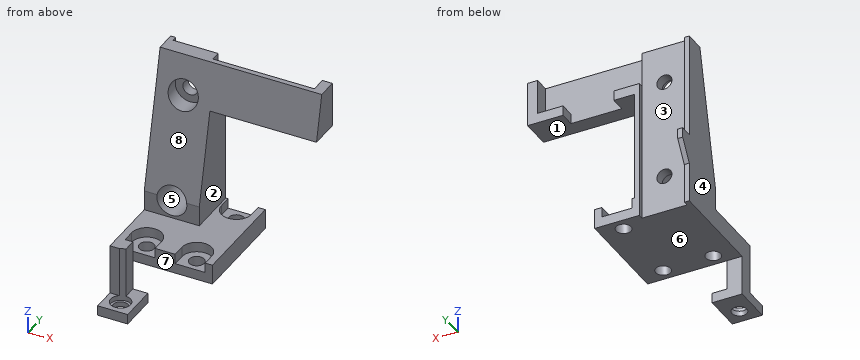
from build123d import *

# Parameters (mm, degrees)
SKETCH_W        = 18.9
SKETCH_H        = 20
SKETCH_R        = 1.5
PAD_DEPTH       = 8
SKETCH001_W     = 3
SKETCH001_H     = 16
PAD001_DEPTH    = 3
SKETCH002_W     = 6
SKETCH002_H     = 7.65
SKETCH002_R     = 1.5
PAD002_DEPTH    = 2
SKETCH003_R     = 2
POCKET_DEPTH    = 15
PAD003_DEPTH    = 10
SKETCH005_R     = 1.5
POCKET001_DEPTH = 10
SKETCH006_W     = 9
SKETCH006_H     = 35
POCKET002_DEPTH = 1
POCKET003_DEPTH = 3
SKETCH008_W     = 1
SKETCH008_H     = 6.05
PAD004_DEPTH    = 2.5
POCKET004_DEPTH = 32.301
POCKET005_DEPTH = 32.301
POCKET014_DEPTH = 6
POCKET015_DEPTH = 4
SKETCH023_R     = 3
POCKET017_DEPTH = 8


with BuildPart() as part:
    # Sketch (on Face6 of Binder) → Pad (new body)
    with BuildSketch(Plane.XY.offset(8)):
        with Locations((14.45, 10)):
            Rectangle(SKETCH_W, SKETCH_H)
        with Locations((19.45, 17.5)):
            Circle(SKETCH_R, mode=Mode.SUBTRACT)
        with Locations((9.45, 2.5)):
            Circle(SKETCH_R, mode=Mode.SUBTRACT)
        with Locations((19.45, 2.5)):
            Circle(SKETCH_R, mode=Mode.SUBTRACT)
    extrude(amount=PAD_DEPTH)

    # Sketch001 (on Face3 of Pad) → Pad001 (join)
    with BuildSketch(Plane.XZ):
        with Locations((6.5, 8)):
            Rectangle(SKETCH001_W, SKETCH001_H)
    extrude(amount=PAD001_DEPTH)

    # Sketch002 (on Face13 of Pad001) → Pad002 (join)
    with BuildSketch(Plane(origin=(0, 0, 0), x_dir=(1, 0, 0), z_dir=(0, 0, -1))):
        with Locations((8, 3.825)):
            Rectangle(SKETCH002_W, SKETCH002_H)
        with Locations((8, 4.65)):
            Circle(SKETCH002_R, mode=Mode.SUBTRACT)
    extrude(amount=-PAD002_DEPTH)

    # Sketch003 (on Face12 of Pad002) → Pocket (cut)
    with BuildSketch(Plane.XY.offset(16)):
        with Locations((8, -4.65)):
            Circle(SKETCH003_R)
    extrude(amount=-POCKET_DEPTH, mode=Mode.SUBTRACT)

    # Sketch004 (on Face1 of Pocket) → Pad003 (join)
    with BuildSketch(Plane(origin=(0, 20, 0), x_dir=(-1, 0, 0), z_dir=(0, 1, 0))):
        Polygon((-5, 16), (-16, 16), (-16, 34.02), (-37.3, 34.02), (-37.3, 43), (-16, 43), (-5, 43), align=None)
    extrude(amount=-PAD003_DEPTH)

    # Sketch005 (on Face5 of Pad003) → Pocket001 (cut)
    with BuildSketch(Plane(origin=(0, 20, 0), x_dir=(-1, 0, 0), z_dir=(0, 1, 0))):
        with Locations((-10.5, 15.5)):
            Circle(SKETCH005_R)
        with Locations((-10.5, 35.5)):
            Circle(SKETCH005_R)
    extrude(amount=-POCKET001_DEPTH, mode=Mode.SUBTRACT)

    # Sketch006 (on Face5 of Pocket001) → Pocket002 (cut)
    with BuildSketch(Plane(origin=(0, 20, 0), x_dir=(-1, 0, 0), z_dir=(0, 1, 0))):
        with Locations((-10.5, 25.5)):
            Rectangle(SKETCH006_W, SKETCH006_H)
    extrude(amount=-POCKET002_DEPTH, mode=Mode.SUBTRACT)

    # Sketch007 (on Face21 of Pocket002) → Pocket003 (cut)
    with BuildSketch(Plane(origin=(0, 20, 0), x_dir=(-1, 0, 0), z_dir=(0, 1, 0))):
        Polygon((-15, 43), (-35.3, 43), (-35.3, 36.02), (-30.23, 36.02), (-30.23, 34.02), (-20.07, 34.02), (-20.07, 36.02), (-15, 36.02), align=None)
    extrude(amount=-POCKET003_DEPTH, mode=Mode.SUBTRACT)

    # Sketch008 (on Face4 of Pocket003) → Pad004 (join)
    with BuildSketch(Plane(origin=(0, 20, 0), x_dir=(-1, 0, 0), z_dir=(0, 1, 0))):
        with Locations((-5.5, 19.025)):
            Rectangle(SKETCH008_W, SKETCH008_H)
    extrude(amount=PAD004_DEPTH)

    # Sketch009 (on Face18 of Pad004) → Pocket004 (cut, through all)
    with BuildSketch(Plane(origin=(5, 0, 0), x_dir=(0, -1, 0), z_dir=(-1, 0, 0))):
        Polygon((-22.5, 20.05), (-20, 16), (-22.5, 16), align=None)
    extrude(amount=-POCKET004_DEPTH, mode=Mode.SUBTRACT)

    # Sketch010 (on Face22 of Pocket004) → Pocket005 (cut, through all)
    with BuildSketch(Plane(origin=(5, 0, 0), x_dir=(0, -1, 0), z_dir=(-1, 0, 0))):
        Polygon((-10, 16), (-16, 43), (-10, 43), align=None)
    extrude(amount=-POCKET005_DEPTH, mode=Mode.SUBTRACT)

    # Sketch020 (on Face21 of Pocket005) → Pocket014 (cut)
    with BuildSketch(Plane.XY.offset(16)):
        with BuildLine():
            ThreePointArc((16.45, 17.499996), (19.45, 14.5), (22.45, 17.499996))
            Line((22.45, 17.499996), (22.45, 20))
            Line((22.45, 20), (16.45, 20))
            Line((16.45, 20), (16.45, 17.499996))
        make_face()
        with BuildLine():
            ThreePointArc((22.45, 2.5), (19.45, 5.5), (16.45, 2.5))
            Line((16.45, 0), (16.45, 2.5))
            Line((22.45, 0), (16.45, 0))
            Line((22.45, 2.5), (22.45, 0))
        make_face()
        with BuildLine():
            ThreePointArc((12.45, 2.5), (9.45, 5.5), (6.45, 2.5))
            Line((6.45, 2.5), (6.45, 0))
            Line((6.45, 0), (12.45, 0))
            Line((12.45, 0), (12.45, 2.5))
        make_face()
    extrude(amount=-POCKET014_DEPTH, mode=Mode.SUBTRACT)

    # Sketch021 (on Face21 of Pocket014) → Pocket015 (cut)
    with BuildSketch(Plane.XY.offset(16)):
        Polygon((23.9, 0), (23.9, 10), (23.9, 20), (16, 20), (16, 10), (5, 10), (5, 0), (5, -3), (8, -3), (8, 0), align=None)
    extrude(amount=-POCKET015_DEPTH, mode=Mode.SUBTRACT)

    # Sketch023 (on Face6 of Pocket015) → Pocket017 (cut)
    with BuildSketch(Plane(origin=(0, 9, 0), x_dir=(-1, 0, 0), z_dir=(0, 1, 0))):
        with Locations((-10.5, 15.5)):
            Circle(SKETCH023_R)
        with Locations((-10.5, 35.5)):
            Circle(SKETCH023_R)
    extrude(amount=POCKET017_DEPTH, mode=Mode.SUBTRACT)


solid = part.part
Work out the finished part from the listing and answer in its coordinate system (mm). Face numbers are marked on the shaded views. A direction names the side the tool comes from. Coordinates: 2 decimals unless noted, no trailing zeros. Write each loop counter-clockwise with the first axis right and the second up, starting at its lowest first coordinate (ties: lowest second). Pieces come first, ordered by that corner, then holes. Notation, with made-up numbers: M -14,-32 L -4,-32 A12 ccw -4,-13 Z; hole C 13.5,14 d10. An arc over 180 degrees is marked long. Write item = value, one per line.
1. Determine the mould class of the marked faces 1, 2, 3 and 4 for opening direction X: released by +X, released by -X, zero draft, split by the parting line, or undercut.
Solution:
face_1 = zero draft
face_2 = released by +X
face_3 = undercut
face_4 = released by -X
2. For the marked faces 5, 6, 7 and 8, determine the directions among +Z, -Z, +X, -X, +Y, -Y from which every point of the face is accessible in a straight line to the end or side of a thin tool.
Solution:
face_5 = -Y
face_6 = -Z, +X, -X, +Y
face_7 = +Z, +X, -Y
face_8 = +Z, +X, -X, -Y
3. The part is cut by section D-D (x = 34.5). Determine the outline of the cut face in (y, z), then the cut area to 3 significant figures.
Solution:
outline = M 14,34.02 L 20,34.02 L 20,36.02 L 17,36.02 L 17,43 L 16,43 Z
area = 23.9 mm2
4. The part is cut by section B-B (y = -4.65). Determine the outline of the cut face in (x, z), then the cut area to 3 significant figures.
Solution:
outline = M 5,0 L 6.5,0 L 6.5,1 L 6,1 L 6,2 L 5,2 Z; M 9.5,0 L 11,0 L 11,2 L 10,2 L 10,1 L 9.5,1 Z
area = 5.00 mm2
5. The part is cut by section C-C (z = 15.5). Determine the outline of the cut face in (x, y).
Solution:
outline = M 5,10 L 7.5,10 L 7.5,17 L 9,17 L 9,19 L 6,19 L 6,20 L 5,20 Z; M 12,17 L 13.5,17 L 13.5,10 L 16,10 L 16,20 L 15,20 L 15,19 L 12,19 Z
6. Straight lines are drawn through the part: line 1 (Z direction, x = 10.5, y = 18.5); line 2 (Y direction, x = 19.45, z = 9.05); line 3 (X direction, y = -4.65, z = 0.6). For each, find the intervals that lie inside material, in ascending order. Write a range as from..to.
Solution:
line_1 = 8..14, 17..34, 37..43
line_2 = 0..1, 4..16, 19..20
line_3 = 5..6.5, 9.5..11
7. Flat-ended cylindrical pins translate along their axes: pin 1 (3 mm diameter, centred on y = -1, z = 9.5, fed in from +X); pin 2 (4.5 mm diameter, centred on x = 26, z = 40.5, fed in from +Y); pin 3 (2.5 mm diameter, centred on x = 12.5, z = 29.5, fed in from +Y). Find the tip coordinate at first contact, or state that the pin passes through.
Solution:
pin_1 = 23.9
pin_2 = 17
pin_3 = 19
8. The part is cut by section A-A (x = 19.45). Determine the outline of the cut face in (y, z).
Solution:
outline = M 0,8 L 1,8 L 1,10 L 0,10 Z; M 4,8 L 16,8 L 16,10 L 14.5,10 L 14.5,12 L 5.5,12 L 5.5,10 L 4,10 Z; M 14,34.02 L 20,34.02 L 20,36.02 L 17,36.02 L 17,43 L 16,43 Z; M 19,8 L 20,8 L 20,10 L 19,10 Z
